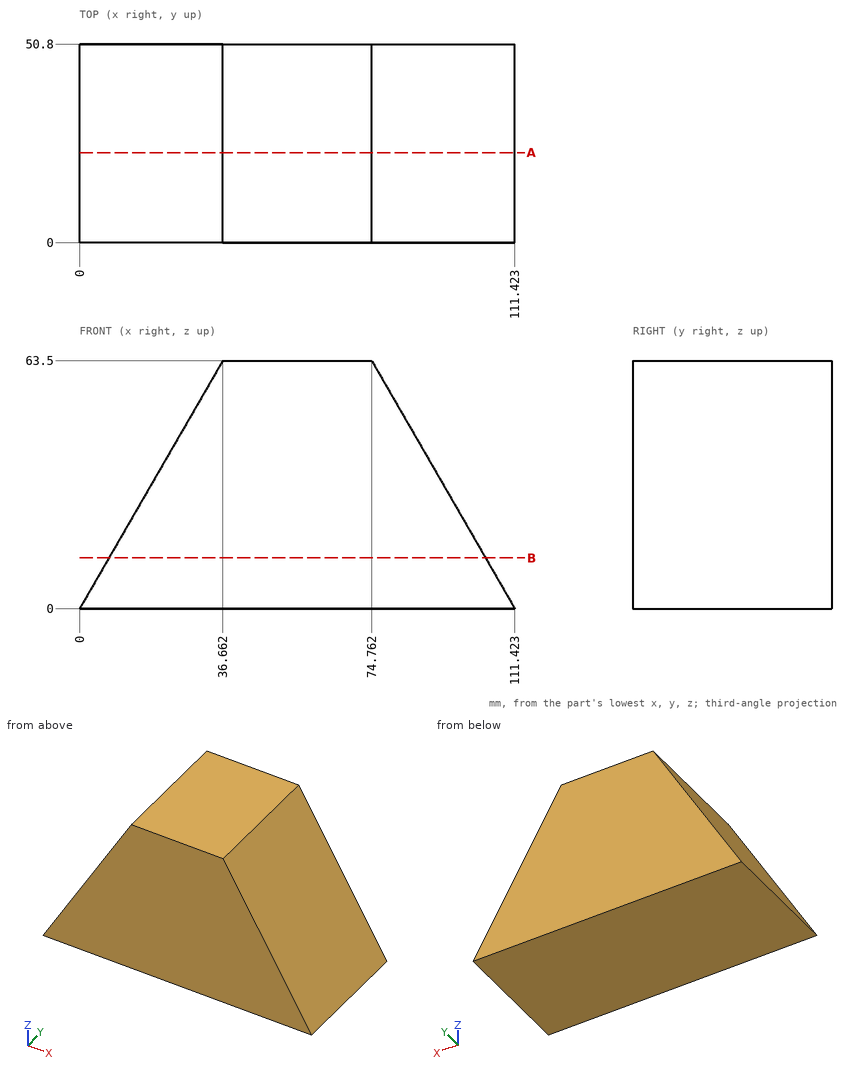
For this review, use the dimensioned drawing (mm, ordinates from the lowest corner) and the shaded views. Round coordinates to 2 decimals unless told otherwise and drop trailing zeros. Write each loop counter-clockwise with the first axis right and the second up, starting at its lowest first coordinate (ties: lowest second). Pieces come first, ordered by that corner, then holes. Notation, with made-up numbers: (75, 65) -> (131, 65) arc R35 ccw to (131, 97) -> close; hole circle Ø2 at (23, -40). An arc over 180 degrees is marked (long way). Use one line per item in the form item = value.
Q1. To check wall thickness, follow probe 1 along X at (y, z) = (25.5, 7.5) (1 decimal); probe 2 along X at (y, z) = (19.5, 21) (1 decimal); probe 3 along Z at (x, y) = (36.5, 35). State the ranges of each line that lie inside material, in increasing order. Write a range as from..to.
Resolved:
probe_1 = 4.3..107.1
probe_2 = 12.1..99.3
probe_3 = 0..63.22
Q2. Consider section B-B (z = 13). State the section outline as (x, y) points (1 decimal), then the cut area to 3 significant figures.
Resolved:
outline = (7.5, 0) -> (103.9, 0) -> (103.9, 50.8) -> (7.5, 50.8) -> close
area = 4,900 mm²
Q3. Consider section A-A (y = 23). State the section outline as (x, z) points, then the cut area to 3 significant figures.
Resolved:
outline = (0, 0) -> (111.42, 0) -> (74.76, 63.5) -> (36.66, 63.5) -> close
area = 4,750 mm²
Q4. Clearance check with flat-ended pins moving along their axes: pin 1 Ø1.5 at (y, z) = (35, 50) entering from -X (1 decimal); pin 2 Ø1 at (y, z) = (12, 41) entering from +X; pin 3 Ø5 at (y, z) = (19.5, 53) entering from -X (1 decimal). State where each tip first meets the part, or that it passes through.
Resolved:
pin_1 = 28.4
pin_2 = 88.04
pin_3 = 29.2
